CAD build for the part. Positions are in the model's coordinates, mm. A direction names the side the tool comes from. Round coordinates to 2 decimals unless told otherwise and drop trailing zeros. Loops run counter-clockwise (first coordinate to the right, second up) from the corner with the lowest first, then second, coordinate; pieces in that order, holes last.
from build123d import *

# Parameters (mm, degrees)
SKETCH1_W                = 50
SKETCH1_H                = 40
BOSS_EXTRUDE1_DEPTH      = 50
CUT_EXTRUDE1_DEPTH       = 69.738635424
SHELL1_T                 = -5
M5_CLEARANCE_HOLE1_D     = 5.5
M5_CLEARANCE_HOLE1_DEPTH = 12
M5_CLEARANCE_HOLE1_TIP   = 1.652366702
CUT_EXTRUDE2_DEPTH       = 1
CUT_EXTRUDE3_DEPTH       = 1
CUT_EXTRUDE4_DEPTH       = 69.738635424
FILLET2_R                = 6
M5_CLEARANCE_HOLE2_D     = 5.5
M5_CLEARANCE_HOLE2_DEPTH = 12
M5_CLEARANCE_HOLE2_TIP   = 1.652366702
BOSS_EXTRUDE2_DEPTH      = 2
BOSS_EXTRUDE2_DEPTH_BACK = 2


with BuildPart() as part:
    # Sketch1 → Boss-Extrude1 (new body)
    with BuildSketch(Plane(origin=(0, 0, 0), x_dir=(1, 0, 0), z_dir=(0, 1, 0))):
        Rectangle(SKETCH1_W, SKETCH1_H)
    extrude(amount=BOSS_EXTRUDE1_DEPTH)

    # Sketch2 → Cut-Extrude1 (cut, through all)
    with BuildSketch(Plane.XY.offset(20)):
        Polygon((-25, 0), (25, 50), (-25, 50), align=None)
    extrude(amount=-CUT_EXTRUDE1_DEPTH, mode=Mode.SUBTRACT)

    # Shell1
    shell1_openings = [part.faces().sort_by_distance(p)[0] for p in [
        (0, 25, 0),
    ]]
    offset(amount=SHELL1_T, openings=shell1_openings, kind=Kind.INTERSECTION)

    # M5 Clearance Hole1
    with Locations(Plane.ZY.offset(-20)):
        with Locations((-10, 38), (-10, 13), (10, 13), (10, 38)):
            Hole(M5_CLEARANCE_HOLE1_D / 2, depth=M5_CLEARANCE_HOLE1_DEPTH)
            with Locations((0, 0, -(M5_CLEARANCE_HOLE1_DEPTH + M5_CLEARANCE_HOLE1_TIP / 2))):  # 118° drill point
                Cone(0, M5_CLEARANCE_HOLE1_D / 2, M5_CLEARANCE_HOLE1_TIP, mode=Mode.SUBTRACT)

    # Sketch5 → Cut-Extrude2 (cut)
    with BuildSketch(Plane.XY.offset(-15)):
        Polygon((-20, 5), (20, 5), (20, 45), align=None)
    extrude(amount=-CUT_EXTRUDE2_DEPTH, mode=Mode.SUBTRACT)

    # Sketch6 → Cut-Extrude3 (cut)
    with BuildSketch(Plane(origin=(0, 0, 15), x_dir=(-1, 0, 0), z_dir=(0, 0, -1))):
        Polygon((-20, 45), (-20, 5), (20, 5), align=None)
    extrude(amount=-CUT_EXTRUDE3_DEPTH, mode=Mode.SUBTRACT)

    # Sketch7 → Cut-Extrude4 (cut, through all)
    with BuildSketch(Plane.XY.offset(20)):
        Polygon((-22.5, 2.5), (-22.5, 0), (-25, 0), align=None)
        Polygon((22.5, 47.5), (25, 47.5), (25, 50), align=None)
    extrude(amount=-CUT_EXTRUDE4_DEPTH, mode=Mode.SUBTRACT)

    # Fillet2
    fillet2_edges = [part.edges().sort_by_distance(p)[0] for p in [
        (-22.5, 2.5, 0),
        (22.5, 47.5, 0),
    ]]
    fillet(fillet2_edges, radius=FILLET2_R)

    # M5 Clearance Hole2
    with Locations(Plane(origin=(0, 5, 0), x_dir=(1, 0, 0), z_dir=(0, 1, 0))):
        with Locations((12, 10), (12, -10), (-13, 10), (-13, -10)):
            Hole(M5_CLEARANCE_HOLE2_D / 2, depth=M5_CLEARANCE_HOLE2_DEPTH)
            with Locations((0, 0, -(M5_CLEARANCE_HOLE2_DEPTH + M5_CLEARANCE_HOLE2_TIP / 2))):  # 118° drill point
                Cone(0, M5_CLEARANCE_HOLE2_D / 2, M5_CLEARANCE_HOLE2_TIP, mode=Mode.SUBTRACT)

    # Sketch10 → Boss-Extrude2 (add, two sides: drawn at the far end of the back side and taken through both)
    with BuildSketch(Plane.XY.offset(-BOSS_EXTRUDE2_DEPTH_BACK)):
        Polygon((20, 45), (20, 5), (-20, 5), align=None)
    extrude(amount=BOSS_EXTRUDE2_DEPTH + BOSS_EXTRUDE2_DEPTH_BACK)


solid = part.part
Item 1: 3-axis set-ups, long thin cutter, end or side, ignore diameter. For faces 1 (the flat face through (6, 18, 20)), 2 (the flat face through (0, 5, -9)): which of +Z, -Z, +X, -X, +Y, -Y reach the whole face in a straight line?
Verdict:
face 1: +Z, +X, -X, +Y, -Y
face 2: -X, +Y
Item 2: Flat gauge pins, fed straight in: P1, Ø2, axis at x = 6, y = 32.5, coming from the -Z side; P2, Ø9, axis at x = 12, z = -10, coming from the -Y side; P3, Ø4, axis at y = 18.5, z = -9.5, coming from the -X side; P4, Ø5, axis at x = -13, z = -0.5, coming from the +Y side. Where does each tip first touch, or does it go through?
Verdict:
P1: passes through
P2: stops at y = 0
P3: stops at x = 20
P4: stops at y = 14.5
Item 3: Mould opens along X. For faces 3 (the cylindrical face through (9.38, 2.46, 9.17)), 4 (the flat face through (-1.6, 23.4, 1.6)), 5 (the flat face through (1, 0, 0)) say: released by +X, released by -X, zero draft, split by the parting line, or undercut.
Verdict:
face 3: undercut
face 4: released by -X
face 5: zero draft
Item 4: Cut at B-B (x = -13). List the corners of the cut face in (y, z).
Verdict:
outline: (0, -20) - (12, -20) - (12, -16) - (5, -16) - (5, -12.75) - (0, -12.75) - close; (0, -7.25) - (5, -7.25) - (5, -2) - (12, -2) - (12, 2) - (5, 2) - (5, 7.25) - (0, 7.25) - close; (0, 12.75) - (5, 12.75) - (5, 16) - (12, 16) - (12, 20) - (0, 20) - close
Item 5: Wall check: L1, parallel to Z at x = -13, y = 2; L2, parallel to Z at x = 0.5, y = 23.5; L3, parallel to Y at x = 21, z = -10. Give the ranges that are in metal, low to high.
Verdict:
L1: z = -20 to -12.75, -7.25 to 7.25, 12.75 to 20
L2: z = -20 to -16, -2 to 2, 16 to 20
L3: y = 0 to 10.25, 15.75 to 35.25, 40.75 to 45.99
Item 6: Cut at C-C (z = -10). State how many separate pieces and enclosed holes the cut face has, plus the area to 3 significant figures.
Verdict:
separate pieces: 5
enclosed holes: 0
area: 332 mm2
Item 7: Cut at A-A (y = 13). List the corners of the cut face in (x, z), plus the area to 3 significant figures.
Verdict:
outline: (-12, -20) - (25, -20) - (25, -12.75) - (20, -12.75) - (20, -16) - (-12, -16) - close; (-12, -2) - (20, -2) - (20, -7.25) - (25, -7.25) - (25, 7.25) - (20, 7.25) - (20, 2) - (-12, 2) - close; (-12, 16) - (20, 16) - (20, 12.75) - (25, 12.75) - (25, 20) - (-12, 20) - close
area: 529 mm2
